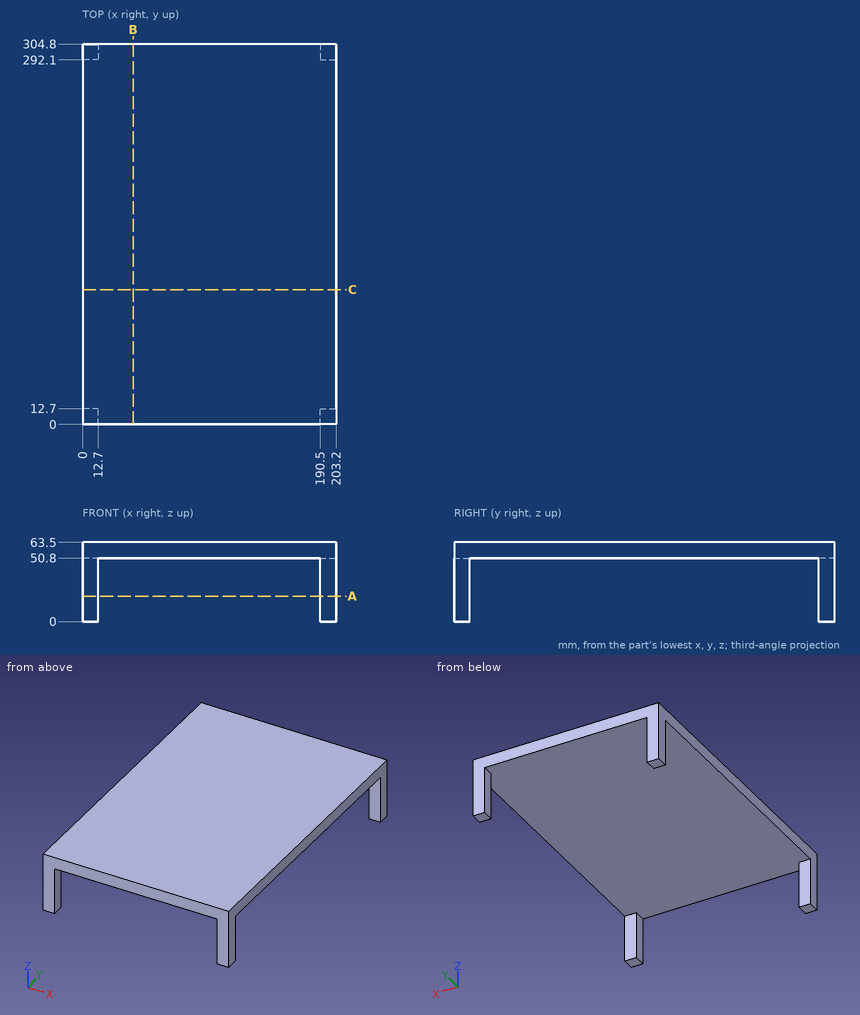
Could you check a few things on this drawing? It's one solid part, dimensions in mm from its lowest x, y, z. Coordinates: 2 decimals unless noted, no trailing zeros. Loops run counter-clockwise (first coordinate to the right, second up) from the corner with the lowest first, then second, coordinate; pieces in that order, holes last. Notation, with made-up numbers: (6.5, -36) - (24.5, -36) arc R13 ccw to (24.5, -21) - close; hole circle Ø4 at (54.25, 18.5). An arc over 180 degrees is marked (long way). Answer as a JSON object with one key per item and string values. Group by question number.
Item 1: If we section it at A-A (z = 20.5): List the corners of the cut face in (x, y) for me.
Item 2: If I drill on L1, parallel to Y at x = 8.5, z = 35.5; L2, parallel to Z at x = 101.5, y = 62.5, over which ranges is the centre line in solid material (lowest first)? Write a range as from..to.
Item 3: If we section it at C-C (y = 108): List the corners of the cut face in (x, z) for me.
Item 4: For pin 1 (2 mm diameter, centred on x = 66, y = 216.5, fed in from -Z); pin 2 (6.5 mm diameter, centred on y = 6, z = 35, fed in from -X), each with a flat end and sliding along its axis, tell me the tip position at first contact or that it passes through.
Item 5: If we section it at B-B (x = 40.5): List the corners of the cut face in (y, z) for me.
Returned:
{
 "1": {"outline": "(0, 0) - (12.7, 0) - (12.7, 12.7) - (0, 12.7) - close; (0, 292.1) - (12.7, 292.1) - (12.7, 304.8) - (0, 304.8) - close; (190.5, 0) - (203.2, 0) - (203.2, 12.7) - (190.5, 12.7) - close; (190.5, 292.1) - (203.2, 292.1) - (203.2, 304.8) - (190.5, 304.8) - close"},
 "2": {"L1": "y = 0..12.7, 292.1..304.8", "L2": "z = 50.8..63.5"},
 "3": {"outline": "(0, 50.8) - (203.2, 50.8) - (203.2, 63.5) - (0, 63.5) - close"},
 "4": {"pin 1": "stops at z = 50.8", "pin 2": "stops at x = 0"},
 "5": {"outline": "(0, 50.8) - (304.8, 50.8) - (304.8, 63.5) - (0, 63.5) - close"}
}
